The listing builds one solid part. Answer for the finished solid, in the listing's coordinates (mm). Face numbers are marked on the shaded views. A direction names the side the tool comes from. Coordinates: 2 decimals unless noted, no trailing zeros. Loops run counter-clockwise (first coordinate to the right, second up) from the corner with the lowest first, then second, coordinate; pieces in that order, holes last. Notation, with made-up numbers: (77, 16.25) - (82, 16.25) arc R10 cw to (82, 24.25) - close; hole circle Ø11 at (22.25, 28.5). An arc over 180 degrees is marked (long way). Use one line per item in the form item = value. Start each with the question number.
```python
from build123d import *

# Parameters (mm, degrees)
F1_DEPTH = 25.4


with BuildPart() as f1:
    # F0 (on Right) → F1 (new body)
    with BuildSketch(Plane.YZ):
        Polygon((-71.3536882989, -62.8876967296), (69.0008763145, -62.8876967296), (69.0008763145, -53.3263756652), (56.4674834127, -53.3263756652), (56.4674834127, -44.460722529), (3.5255327821, -44.460722529), (-3.5255327821, -44.460722529), (-56.4674834127, -44.460722529), (-56.4674834127, -53.3263756652), (-71.3536882989, -53.3263756652), align=None)
        Polygon((-3.5255327821, -44.460722529), (3.5255327821, -44.460722529), (3.5255327821, -36.7242954671), (3.5255327821, -33.3946272731), (3.5255327821, -22.8180289268), (3.5255327821, -19.6842234582), (3.5255327821, -11.2621178851), (3.5255327821, -6.7572705448), (3.5255327821, 0), (3.5255327821, 2.6441493537), (3.5255327821, 55.5271357298), (3.5255327821, 65.5161440372), (-3.5255327821, 65.5161440372), (-3.5255327821, 55.5271357298), (-3.5255327821, 2.6441493537), (-3.5255327821, 0), (-3.5255327821, -6.7572705448), (-3.5255327821, -11.2621178851), (-3.5255327821, -19.096635282), (-3.5255327821, -22.8180289268), (-3.5255327821, -33.3946272731), (-3.5255327821, -36.7242954671), align=None)
        with BuildLine():
            Line((3.5255327821, -33.3946272731), (3.5255327821, -36.7242954671))
            add(Edge.make_bspline(
                [(3.5255327821, -36.7242954671), (19.5283458683, -37.9115714543), (46.0250919066, -39.8774102191), (57.086801682, -19.6662649434), (60.7679214598, 25.1450505181), (63.2637217641, 55.5271357298)],
                knots=[0, 0, 0, 0, 0.3293254758, 0.5452824731, 1, 1, 1, 1], degree=3))
            Line((63.2637217641, 55.5271357298), (59.542324394, 55.5271357298))
            add(Edge.make_bspline(
                [(59.542324394, 55.5271357298), (55.0176134141, 25.2060017822), (48.567756102, -18.0159826428), (42.1295842811, -35.83733265), (18.2774691458, -34.3280690461), (3.5255327821, -33.3946272731)],
                knots=[0, 0, 0, 0, 0.4727701883, 0.6739215543, 1, 1, 1, 1], degree=3))
        make_face()
        with BuildLine():
            add(Edge.make_bspline(
                [(-3.5255327821, -36.7242954671), (-24.2986218761, -37.8725969995), (-58.7436757829, -39.7766618214), (-61.2954694033, -9.4828326596), (-62.0184453958, 30.5452331605), (-62.4802745879, 56.1147257686)],
                knots=[0, 0, 0, 0, 0.3543477365, 0.5875643641, 1, 1, 1, 1], degree=3))
            Line((-3.5255327821, -36.7242954671), (-3.5255327821, -33.3946272731))
            add(Edge.make_bspline(
                [(-58.9547343552, 56.1147257686), (-58.5518682204, 23.6575228224), (-57.9849643897, -22.0154963092), (-44.9012456447, -34.1194273047), (-19.6651093216, -33.677352688), (-3.5255327821, -33.3946272731)],
                knots=[0, 0, 0, 0, 0.469569513, 0.6607672691, 1, 1, 1, 1], degree=3))
            Line((-58.9547343552, 56.1147257686), (-62.4802745879, 56.1147257686))
        make_face()
        with BuildLine():
            Line((3.5255327821, -19.6842234582), (3.5255327821, -22.8180289268))
            add(Edge.make_bspline(
                [(3.5255327821, -22.8180289268), (15.0074258417, -26.1390970683), (45.1615775397, -34.8610031178), (48.4786261835, 21.0817469198), (50.5326315761, 55.7229965925)],
                knots=[0, 0, 0, 0, 0.3807732074, 1, 1, 1, 1], degree=3))
            Line((50.5326315761, 55.7229965925), (46.6153733432, 55.7229965925))
            add(Edge.make_bspline(
                [(46.6153733432, 55.7229965925), (44.908074699, 27.2957561446), (42.3414520643, -15.4395901418), (19.7553258166, -24.281474601), (8.8547514125, -21.1937779169), (3.5255327821, -19.6842234582)],
                knots=[0, 0, 0, 0, 0.5038360705, 0.757428741, 1, 1, 1, 1], degree=3))
        make_face()
        with BuildLine():
            add(Edge.make_bspline(
                [(-3.5255327821, -22.8180289268), (-16.4749058597, -26.1817426868), (-49.3027052775, -34.7090528466), (-48.9708309091, 21.6160802328), (-48.7698689103, 55.7229965925)],
                knots=[0, 0, 0, 0, 0.3944636347, 1, 1, 1, 1], degree=3))
            Line((-3.5255327821, -22.8180289268), (-3.5255327821, -19.096635282))
            add(Edge.make_bspline(
                [(-43.4815697372, 55.7229965925), (-43.1493925226, 27.3035954994), (-42.6784250485, -12.9899976808), (-28.0554027813, -20.855813996), (-12.619326686, -19.7488037879), (-3.5255327821, -19.096635282)],
                knots=[0, 0, 0, 0, 0.4958091065, 0.7029680312, 1, 1, 1, 1], degree=3))
            Line((-43.4815697372, 55.7229965925), (-48.7698689103, 55.7229965925))
        make_face()
        with BuildLine():
            Line((3.5255327821, -6.7572705448), (3.5255327821, -11.2621178851))
            add(Edge.make_bspline(
                [(3.5255327821, -11.2621178851), (11.5964613447, -13.5255916132), (34.0307157026, -19.8172276939), (35.8520182308, 26.356535863), (37.0180904865, 55.9188649058)],
                knots=[0, 0, 0, 0, 0.3597591627, 1, 1, 1, 1], degree=3))
            Line((37.0180904865, 55.9188649058), (32.904971391, 55.9188649058))
            add(Edge.make_bspline(
                [(32.904971391, 55.9188649058), (32.383994158, 28.9003589611), (31.6256536405, -10.4280924226), (11.0670405767, -8.8444018794), (5.8199367134, -7.3922526292), (3.5255327821, -6.7572705448)],
                knots=[0, 0, 0, 0, 0.5525942812, 0.8043626605, 1, 1, 1, 1], degree=3))
        make_face()
        with BuildLine():
            add(Edge.make_bspline(
                [(-3.5255327821, -11.2621178851), (-13.9628252189, -13.979458265), (-40.9413722155, -21.0033004721), (-36.6880011003, 26.4390107496), (-34.0801477432, 55.5271357298)],
                knots=[0, 0, 0, 0, 0.3868737793, 1, 1, 1, 1], degree=3))
            Line((-3.5255327821, -11.2621178851), (-3.5255327821, -6.7572705448))
            add(Edge.make_bspline(
                [(-30.1628876477, 55.5271357298), (-31.985444285, 30.8578224877), (-34.5222487441, -3.4792305049), (-23.1181589343, -10.8027369268), (-10.8430847617, -8.2681915567), (-3.5255327821, -6.7572705448)],
                knots=[0, 0, 0, 0, 0.5075246544, 0.7064201903, 1, 1, 1, 1], degree=3))
            Line((-30.1628876477, 55.5271357298), (-34.0801477432, 55.5271357298))
        make_face()
        with BuildLine():
            Line((3.5255327821, 2.6441493537), (3.5255327821, 0))
            add(Edge.make_bspline(
                [(3.5255327821, 0), (8.5496923219, -1.4975662301), (23.8660891446, -6.0629703473), (24.703557743, 31.1252007713), (25.266315788, 56.1147257686)],
                knots=[0, 0, 0, 0, 0.3280249002, 1, 1, 1, 1], degree=3))
            Line((25.266315788, 56.1147257686), (20.3697439283, 56.1147257686))
            add(Edge.make_bspline(
                [(20.3697439283, 56.1147257686), (20.8792514929, 35.723351714), (21.6022738177, 6.7867476282), (10.2200746725, 1.8146451795), (5.6493055923, 2.3809979029), (3.5255327821, 2.6441493537)],
                knots=[0, 0, 0, 0, 0.5609253817, 0.7959873449, 1, 1, 1, 1], degree=3))
        make_face()
        with BuildLine():
            add(Edge.make_bspline(
                [(-3.5255327821, 0), (-8.5619762859, -1.4869958031), (-23.9379763758, -6.0267166565), (-22.6242184339, 31.0121575033), (-21.7407848686, 55.9188649058)],
                knots=[0, 0, 0, 0, 0.3275522551, 1, 1, 1, 1], degree=3))
            Line((-3.5255327821, 0), (-3.5255327821, 2.6441493537))
            add(Edge.make_bspline(
                [(-16.8442111462, 55.9188649058), (-18.1566177579, 33.0480107342), (-19.8170856078, 4.1116142591), (-13.5367557364, 2.8459613048), (-7.3849929996, 2.7219505575), (-3.5255327821, 2.6441493537)],
                knots=[0, 0, 0, 0, 0.5842044945, 0.7391404252, 1, 1, 1, 1], degree=3))
            Line((-16.8442111462, 55.9188649058), (-21.7407848686, 55.9188649058))
        make_face()
    extrude(amount=F1_DEPTH)


solid = f1.part
```
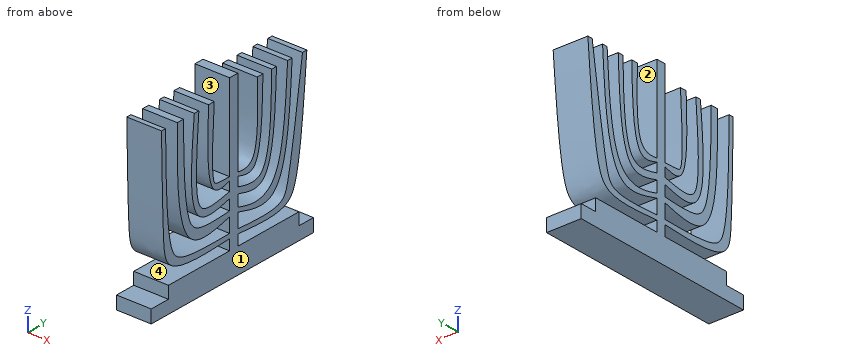
(1) For the marked faces 1 and 2, determine the directions among +Z, -Z, +X, -X, +Y, -Y from which every point of the face is accessible in a straight line to the end or side of a thin tool.
(2) Find the intervals of material crossed by probe 1 along Y at (x, z) = (10.5, -41.5); probe 2 along Z at (x, y) = (5.75, 9); probe 3 along Y at (x, z) = (8.5, -44.5), in increasing order. Write a range as from..to.
(3) A cutting plane is placed at A-A (z = 20.5). State how many separate pieces and enclosed holes the cut face has, then the cut area to 3 significant figures.
(4) A cutting plane is placed at C-C (z = -50.5). Determine the outline of the cut face in (x, y), then the cut area to 3 significant figures.
(5) Each of these flat-tipped pins is pushed along its axis until it touches: pin 1 Ø2 at (x, z) = (20, -21) entering from +Y; pin 2 Ø3 at (x, z) = (10.5, -36.5) entering from +Y; pin 3 Ø6.5 at (x, z) = (9, -14) entering from -Y; pin 4 Ø10 at (x, z) = (16.5, -51) entering from -Y. Where does it stop, or does it pass through?
(6) Determine the mould class of the marked faces 3 and 4 for opening direction Y: +Y half, -Y half, draft (parallel to the pull), parting line (faces both ways), or undercut.
Evaluation:
q1.face_1 = +Z, -Z, +X, +Y, -Y
q1.face_2 = +Z, +X, -X
q2.probe_1 = -3.53..3.53
q2.probe_2 = -62.89..-44.46, -37.12..-33.73, -24.37..-21.16, -12.73..-8.12, -1.43..2.34
q2.probe_3 = -56.47..56.47
q3.separate_pieces = 9
q3.enclosed_holes = 0
q3.area = 1,050 mm^2
q4.outline = (0, -56.47) - (25.4, -56.47) - (25.4, 56.47) - (0, 56.47) - close
q4.area = 2,870 mm^2
q5.pin_1 = 54.38
q5.pin_2 = 45.26
q5.pin_3 = -60.79
q5.pin_4 = -71.35
q6.face_3 = undercut
q6.face_4 = draft
